from build123d import *

# Parameters (mm, degrees)
SKETCH1_R           = 10
BOSS_EXTRUDE1_DEPTH = 3
SKETCH3_R           = 12
BOSS_EXTRUDE2_DEPTH = 0.8
CUT_EXTRUDE1_DEPTH  = 18.390802167
CHAMFER1_SIZE       = 0.4


with BuildPart() as part:
    # Sketch1 → Boss-Extrude1 (new body)
    with BuildSketch(Plane(origin=(0, 0, 0), x_dir=(1, 0, 0), z_dir=(0, 1, 0))):
        with Locations(Location((0, 0, 0), (0, 0, 270))):
            Circle(SKETCH1_R)
        Polygon((0, 2.309401077), (-2, 1.154700538), (-2, -1.154700538), (0, -2.309401077), (2, -1.154700538), (2, 1.154700538), align=None, mode=Mode.SUBTRACT)
    extrude(amount=BOSS_EXTRUDE1_DEPTH)

    # Sketch3 → Boss-Extrude2 (add)
    with BuildSketch(Plane(origin=(0, 3, 0), x_dir=(1, 0, 0), z_dir=(0, 1, 0))):
        with Locations(Location((0, 0, 0), (0, 0, 270))):
            Circle(SKETCH3_R)
    extrude(amount=BOSS_EXTRUDE2_DEPTH)

    # Sketch4 → Cut-Extrude1 (cut, through all)
    with BuildSketch(Plane.XZ):
        Polygon((0, -2.309401077), (2, -1.154700538), (2, 1.154700538), (0, 2.309401077), (-2, 1.154700538), (-2, -1.154700538), align=None)
    extrude(amount=-CUT_EXTRUDE1_DEPTH, mode=Mode.SUBTRACT)

    # Chamfer1
    chamfer1_edges = [part.edges().sort_by_distance(p)[0] for p in [
        (0, 3, -10),
    ]]
    chamfer(chamfer1_edges, length=CHAMFER1_SIZE)


solid = part.part
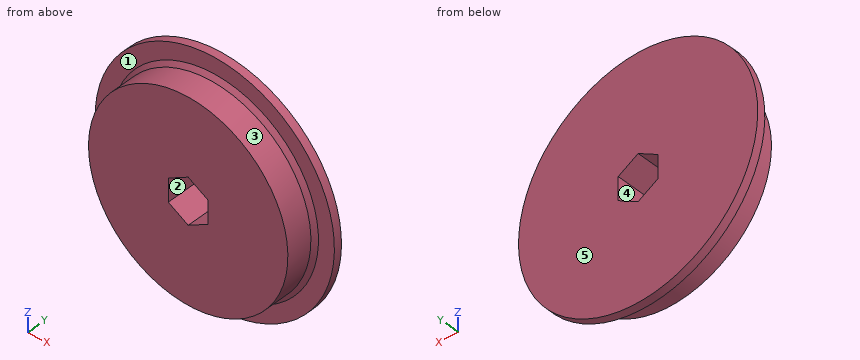
Check sheet for the modelled part. Datum: model origin and axes. Units: mm. Face numbers are marked on the shaded views. A direction names the side the tool comes from. Give positions to 0.01 mm unless a question says otherwise; leave off trailing zeros. Loops run counter-clockwise (first coordinate to the right, second up) from the corner with the lowest first, then second, coordinate; pieces in that order, holes last. Notation, with made-up numbers: M 32,16 L 41,16 A20 cw 41,36 Z; hole C 81,47 d2. An arc over 180 degrees is marked long. Answer as a JSON object with one key per item and string values. Group by question number.
Q1. Go/stop test with flat-tipped pins: P1, Ø8, axis at x = 2.5, z = -7, coming from the -Y side; P2, Ø1, axis at y = 1, z = -9, coming from the +X side; P3, Ø1, axis at y = 2, z = -3, coming from the -X side; P4, Ø1.5, axis at y = 3, z = -4, coming from the +X side. Record where each tip stops, or that it passes through.
Q2. Material ranges on line 1 along X through (y, z) = (3.2, 0.25); line 2 along Y through (x, z) = (-11, -2.25); line 3 along X through (y, z) = (3.2, 2.25), recorded low to high. Write a range as [from, to].
Q3. Cross-section at B-B on y = 0.55. Record the cut outline in (x, z), then the cut area to 3 significant figures.
Q4. Cross-section at C-C on y = 3.45. Record the cut outline in (x, z), then the cut area to 3 significant figures.
Q5. Cross-section at A-A on z = 0. Record the cut outline in (x, y), then the cut area to 3 significant figures.
Q6. Access from +Z, -Z, +X, -X, +Y, -Y to the whole of each face (thin tool, end or side, straight path). Record for the marked faces 4 and 5.
Q7. Release check for a two-part mould opening along X. For the marked faces 1, 2 and 3 record: released by +X, released by -X, zero draft, split by the parting line, or undercut.
Evaluation:
{
 "1": {"P1": "stops at y = 0", "P2": "stops at x = 5.27", "P3": "stops at x = -9.68", "P4": "stops at x = 11.55"},
 "2": {"line 1": "x = [-12, -2], [2, 12]", "line 2": "y = [3, 3.8]", "line 3": "x = [-11.79, -0.1], [0.1, 11.79]"},
 "3": {"outline": "C 0,0 d20; hole M -2,-1.15 L 0,-2.31 L 2,-1.15 L 2,1.15 L 0,2.31 L -2,1.15 Z", "area": "300 mm2"},
 "4": {"outline": "C 0,0 d24; hole M -2,-1.15 L 0,-2.31 L 2,-1.15 L 2,1.15 L 0,2.31 L -2,1.15 Z", "area": "439 mm2"},
 "5": {"outline": "M -12,3 L -10.4,3 L -10,2.6 L -10,0 L -2,0 L -2,3.8 L -12,3.8 Z; M 2,0 L 10,0 L 10,2.6 L 10.4,3 L 12,3 L 12,3.8 L 2,3.8 Z", "area": "64.2 mm2"},
 "6": {"face 4": "+Y, -Y", "face 5": "+Z, -Z, +X, -X, +Y"},
 "7": {"face 1": "zero draft", "face 2": "undercut", "face 3": "split by the parting line"}
}
